Here's how the part is built. I have some questions about the finished solid (model axes, mm). Coordinates: 2 decimals unless noted, no trailing zeros. Write each loop counter-clockwise with the first axis right and the second up, starting at its lowest first coordinate (ties: lowest second). Pieces come first, ordered by that corner, then holes.
Item 1: I want a section at B-B (x = -203.2). Please give me the cut outline in (y, z).
Item 2: I want a section at C-C (x = -64.77). Please give me the cut outline in (y, z), and give its area (3 significant figures).
Item 3: I want a section at D-D (z = 215.9). Please give me the cut outline in (x, y).
Item 4: I want a section at A-A (z = 124.46). Please give me the cut outline in (x, y).
Item 5: If we mould it in two halves opening along X, with no side actions, what happens to faces 1 (the face through (-101, -4.775, 101)), 2 (the face through (-89.95, -2.35, 211.19)), 3 (the face through (-252.09, -2.35, 87.09))? For each: pulls with the +X half, pulls with the -X half, needs draft (parallel to the pull), parting line crosses it, or undercut.
Item 6: Please list where these lines run through material, in increasing order: line 1 (Z direction, x = -207.5, y = -3.2); line 2 (Z direction, x = -205, y = -1.3); line 3 (Z direction, x = -240, y = -1).
Item 7: I'm going to push flat-ended pins straight in: P1, Ø11, axis at x = -203.2, z = 76.2, coming from the -Y side; P2, Ø2.5, axis at x = -149.5, y = -3.5, coming from the +Z side. Where does each tip first touch, or does it pass through?
from build123d import *

# Parameters (mm, degrees)
F0_R     = 4.826
F0_R_2   = 9.525
F0_R_3   = 9.652
F1_DEPTH = 4.7752


with BuildPart() as f1:
    # F0 (on Front) → F1 (new body)
    with BuildSketch(Plane.XZ):
        with BuildLine():
            ThreePointArc((-6.35, 0), (-1.859872, 1.859872), (0, 6.35))
            Line((0, 6.35), (0, 247.65))
            ThreePointArc((0, 247.65), (-1.859872, 252.140128), (-6.35, 254))
            Line((-6.35, 254), (-95.25, 254))
            ThreePointArc((-95.25, 254), (-99.740128, 252.140128), (-101.6, 247.65))
            Line((-101.6, 247.65), (-101.6, 176.188146))
            ThreePointArc((-101.6, 176.188146), (-35.670644, 180.900035), (-1.27, 124.46))
            ThreePointArc((-1.27, 124.46), (-46.17483, 63.743695), (-117.379281, 88.9))
            Line((-117.379281, 88.9), (-247.65, 88.9))
            ThreePointArc((-247.65, 88.9), (-252.140128, 87.040128), (-254, 82.55))
            Line((-254, 82.55), (-254, 6.35))
            ThreePointArc((-254, 6.35), (-252.140128, 1.859872), (-247.65, 0))
            Line((-247.65, 0), (-6.35, 0))
        make_face()
        with Locations((-203.2, 38.1)):
            Circle(F0_R, mode=Mode.SUBTRACT)
        with Locations((-203.2, 76.2)):
            Circle(F0_R, mode=Mode.SUBTRACT)
        with Locations((-33.35242, 48.26)):
            Circle(F0_R_2, mode=Mode.SUBTRACT)
        with Locations((-88.9, 215.9)):
            Circle(F0_R, mode=Mode.SUBTRACT)
        with Locations((-38.1, 215.9)):
            Circle(F0_R, mode=Mode.SUBTRACT)
        with Locations((-7.62, 215.9)):
            Circle(F0_R, mode=Mode.SUBTRACT)
        with Locations((-33.35242, 48.26)):
            Circle(F0_R_2)
        with BuildLine():
            ThreePointArc((-1.27, 124.46), (-35.670644, 180.900035), (-101.6, 176.188146))
            Line((-101.6, 176.188146), (-101.6, 101.6))
            ThreePointArc((-101.6, 101.6), (-105.319744, 92.619744), (-114.3, 88.9))
            Line((-114.3, 88.9), (-117.379281, 88.9))
            ThreePointArc((-117.379281, 88.9), (-46.17483, 63.743695), (-1.27, 124.46))
        make_face()
        with Locations((-64.77, 124.46)):
            Circle(F0_R_3, mode=Mode.SUBTRACT)
    extrude(amount=F1_DEPTH)


solid = f1.part
Answer:
1. outline: (-4.78, 0) - (0, 0) - (0, 33.27) - (-4.78, 33.27) - close; (-4.78, 42.93) - (0, 42.93) - (0, 71.37) - (-4.78, 71.37) - close; (-4.78, 81.03) - (0, 81.03) - (0, 88.9) - (-4.78, 88.9) - close
2. outline: (-4.78, 0) - (0, 0) - (0, 114.81) - (-4.78, 114.81) - close; (-4.78, 134.11) - (0, 134.11) - (0, 254) - (-4.78, 254) - close
2. area: 1,120 mm2
3. outline: (-101.6, -4.78) - (-93.73, -4.78) - (-93.73, 0) - (-101.6, 0) - close; (-84.07, -4.78) - (-42.93, -4.78) - (-42.93, 0) - (-84.07, 0) - close; (-33.27, -4.78) - (-12.45, -4.78) - (-12.45, 0) - (-33.27, 0) - close; (-2.79, -4.78) - (0, -4.78) - (0, 0) - (-2.79, 0) - close
4. outline: (-101.6, -4.78) - (-74.42, -4.78) - (-74.42, 0) - (-101.6, 0) - close; (-55.12, -4.78) - (0, -4.78) - (0, 0) - (-55.12, 0) - close
5. face 1: needs draft
5. face 2: undercut
5. face 3: pulls with the -X half
6. line 1: z = 0 to 35.91, 40.29 to 74.01, 78.39 to 88.9
6. line 2: z = 0 to 33.62, 42.58 to 71.72, 80.68 to 88.9
6. line 3: z = 0 to 88.9
7. P1: stops at y = -4.78
7. P2: stops at z = 88.9
